```python
from build123d import *

# Parameters (mm, degrees)
BOX006_W          = 15
BOX006_H          = 26
BOX006_DEPTH      = 64
CYLINDER023_R     = 15.17
CYLINDER023_DEPTH = 64
BOX005_W          = 40
BOX005_H          = 2
BOX005_DEPTH      = 60
CYLINDER022_R     = 17.17
CYLINDER022_DEPTH = 60


with BuildPart() as cube004:
    # Box006 → Box006 (new body)
    with BuildSketch(Plane(origin=(4, -11, -2), x_dir=(1, 0, 0), z_dir=(0, 0, 1))):
        with Locations((7.5, 13)):
            Rectangle(BOX006_W, BOX006_H)
    extrude(amount=BOX006_DEPTH)


with BuildPart() as fusion002003003009:
    # Cylinder023 → Cylinder023 (new body)
    with BuildSketch(Plane.XY.offset(-2)):
        Circle(CYLINDER023_R)
    extrude(amount=CYLINDER023_DEPTH)

    # Fusion002003003009: union Cube004
    add(cube004.part)


with BuildPart() as cube003:
    # Box005 → Box005 (new body)
    with BuildSketch(Plane(origin=(0, 15, 0), x_dir=(1, 0, 0), z_dir=(0, 0, 1))):
        with Locations((20, 1)):
            Rectangle(BOX005_W, BOX005_H)
    extrude(amount=BOX005_DEPTH)


with BuildPart() as obj1:
    # Cylinder022 → Cylinder022 (new body)
    with BuildSketch(Plane.XY):
        Circle(CYLINDER022_R)
    extrude(amount=CYLINDER022_DEPTH)

    # Fusion002003003010: union Cube003
    add(cube003.part)

    # Cut001011003002: cut Fusion002003003009
    add(fusion002003003009.part, mode=Mode.SUBTRACT)


solid = obj1.part
```
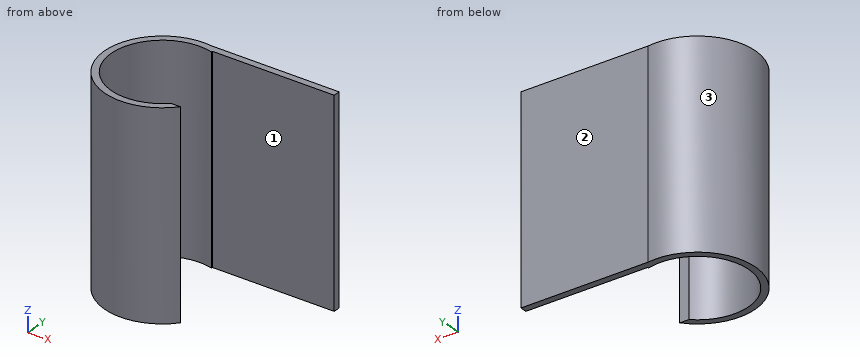
The model under review builds one solid part; all positions refer to its coordinate system, in mm. Face numbers are marked on the shaded views. A direction names the side the tool comes from. Round coordinates to 2 decimals unless told otherwise and drop trailing zeros. Order: outer loops, then holes, each group sorted by start corner. A loop starts at its lowest first (then second) coordinate and runs counter-clockwise, first axis right, second up.
(1) Wall thickness on L1, parallel to Y at x = 0, z = 21; L2, parallel to X at y = 0, z = 24; L3, parallel to Y at x = 25.5, z = 17.5: over which ranges is each line inside the solid? List them lowest first.
Working result:
L1: y = -17.17 to -15.17, 15.17 to 17.17
L2: x = -17.17 to -15.17
L3: y = 15 to 17
(2) Tool access review of the marked faces 1, 2 and 3: name each direction out of +Z, -Z, +X, -X, +Y, -Y from which nothing blocks a thin tool from reaching the whole face with its end or side.
Working result:
face 1: +Z, -Z, +X
face 2: +Z, -Z, +X, +Y
face 3: +Z, -Z
(3) For P1, Ø10, axis at x = 32, z = 38, coming from the -Y side; P2, Ø18, axis at x = 15.5, z = 22, coming from the -Y side; P3, Ø0.8, axis at x = 11.5, z = 16, coming from the +Y side, all flat-tipped, find the tip position at first contact; note any pin that passes through.
Working result:
P1: stops at y = 15
P2: stops at y = -15.89
P3: stops at y = 17
(4) Take a section at B-B, the plane z = 31. State the section outline as (x, y) points, plus the area to 3 significant figures.
Working result:
outline: (2.41, 17) arc R17.17 ccw (long way) to (13.18, -11) - (10.45, -11) arc R15.17 cw (long way) to (4, 14.63) - (4, 15) - (40, 15) - (40, 17) - close
area: 208 mm2
(5) Take a section at C-C, the plane y = -14. State the section outline as (x, z) points, plus the area to 3 significant figures.
Working result:
outline: (-9.94, 0) - (-5.84, 0) - (-5.84, 60) - (-9.94, 60) - close; (5.84, 0) - (9.94, 0) - (9.94, 60) - (5.84, 60) - close
area: 492 mm2
(6) Take a section at D-D, the plane y = 0. State the section outline as (x, z) points, plus the area to 3 significant figures.
Working result:
outline: (-17.17, 0) - (-15.17, 0) - (-15.17, 60) - (-17.17, 60) - close
area: 120 mm2
(7) Take a section at A-A, the plane x = 0. State the section outline as (y, z) points, plus the area to 3 significant figures.
Working result:
outline: (-17.17, 0) - (-15.17, 0) - (-15.17, 60) - (-17.17, 60) - close; (15.17, 0) - (17.17, 0) - (17.17, 60) - (15.17, 60) - close
area: 240 mm2
